Design review of the part shown in the three views and the two pictorial views. Dimensions are in mm from the part's minimum x, y and z. A direction names the side the tool comes from. Give positions to 0.01 mm unless a question says otherwise; leave off trailing zeros. Loops run counter-clockwise (first coordinate to the right, second up) from the corner with the lowest first, then second, coordinate; pieces in that order, holes last. Notation, with made-up numbers: (-35, -31.75) - (-5, -31.75) arc R21 cw to (-5, -9.75) - close; hole circle Ø10 at (-2.75, 36.25). An arc over 180 degrees is marked (long way). Use CSV: the item, a comma, the result in double quotes. Start each with the question number.
1. Mouldability with a two-part tool opening along X and no side actions: class the marked faces 3, 4 and 5 as pulls with the +X half, pulls with the -X half, needs draft (parallel to the pull), parting line crosses it, or undercut.
2. For the marked faces 1 and 2, list the 3-axis set-ups (+Z, -Z, +X, -X, +Y, -Y) from which the entire face can be reached by the end or side of a thin tool; tool diameter is ignored.
3. Take a section at A-A on z = 16. Give the boundary of the cut face in (x, y) (1 decimal).
4. Take a section at D-D on y = 3.25. Give the boundary of the cut face in (x, z) (1 decimal).
5. Take a section at C-C on z = 33. State how many separate pieces and enclosed holes the cut face has, plus the area to 3 significant figures.
6. Wall thickness on line 1 (Z direction, x = 13, y = 11.5); line 2 (Y direction, x = 30, z = 25); line 3 (Z direction, x = 7, y = 4.5): over which ranges is each line inside the solid? List them lowest first.
7. For pin 1 (7.5 mm diameter, centred on x = 26.26, y = 6.03, fed in from -Z); pin 2 (16 mm diameter, centred on x = 14.5, z = 22.5, fed in from -Y), all flat-tipped, find the tip position at first contact; note any pin that passes through.
8. Take a section at B-B on x = 11. Give the boundary of the cut face in (y, z).
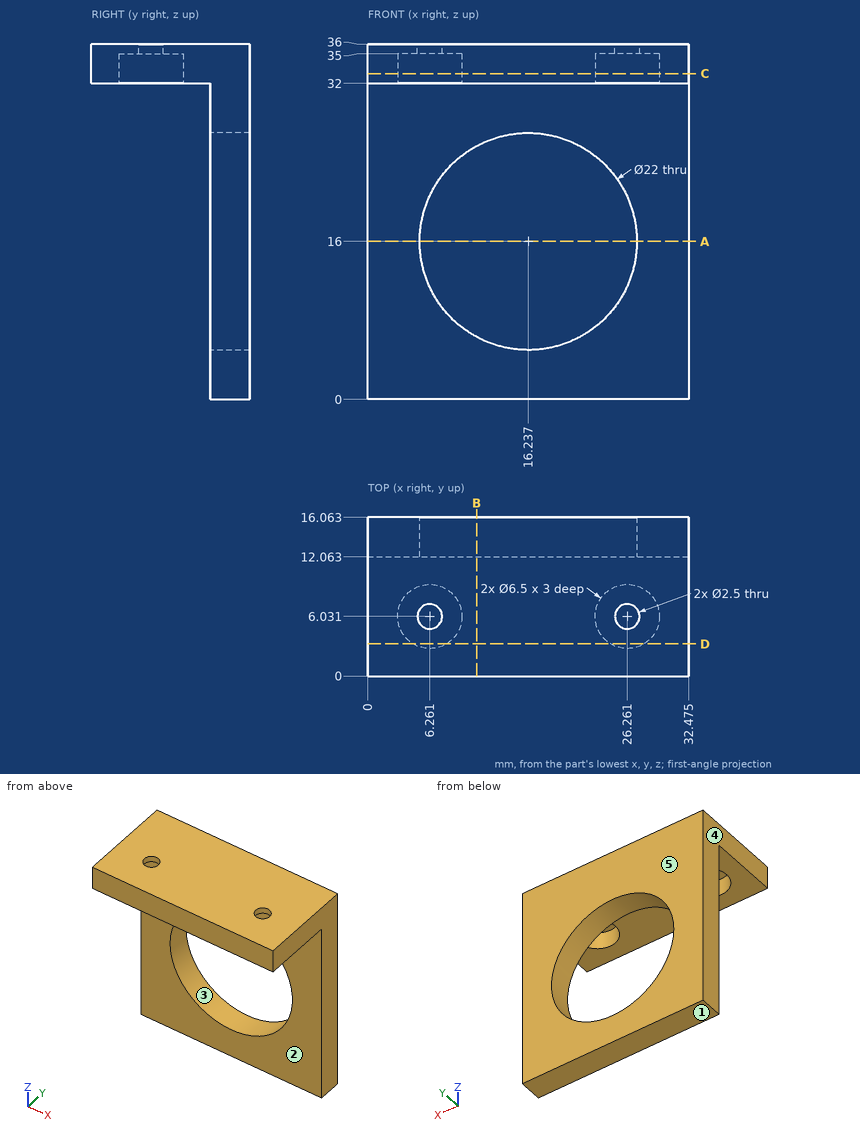
Check result:
1,face 3,"undercut"
1,face 4,"pulls with the -X half"
1,face 5,"needs draft"
2,face 1,"-Z, +X, -X, +Y, -Y"
2,face 2,"-Z, +X, -X, -Y"
3,outline,"(0, 12.1) - (5.2, 12.1) - (5.2, 16.1) - (0, 16.1) - close; (27.2, 12.1) - (32.5, 12.1) - (32.5, 16.1) - (27.2, 16.1) - close"
4,outline,"(0, 32) - (4.6, 32) - (4.6, 35) - (7.9, 35) - (7.9, 32) - (24.6, 32) - (24.6, 35) - (27.9, 35) - (27.9, 32) - (32.5, 32) - (32.5, 36) - (0, 36) - close"
5,separate pieces,"1"
5,enclosed holes,"2"
5,area,"455 mm²"
6,line 1,"z = 32 to 36"
6,line 2,"y = 12.06 to 16.06"
6,line 3,"z = 35 to 36"
7,pin 1,"stops at z = 32"
7,pin 2,"stops at y = 12.06"
8,outline,"(0, 32) - (12.06, 32) - (12.06, 25.67) - (16.06, 25.67) - (16.06, 36) - (0, 36) - close; (12.06, 0) - (16.06, 0) - (16.06, 6.33) - (12.06, 6.33) - close"
